Geometry check sheet. Reference: the model listing, model coordinates, mm. Face numbers are marked on the shaded views. Give positions to 0.01 mm unless a question says otherwise; leave off trailing zeros. Order: outer loops, then holes, each group sorted by start corner. A loop starts at its lowest first (then second) coordinate and runs counter-clockwise, first axis right, second up.
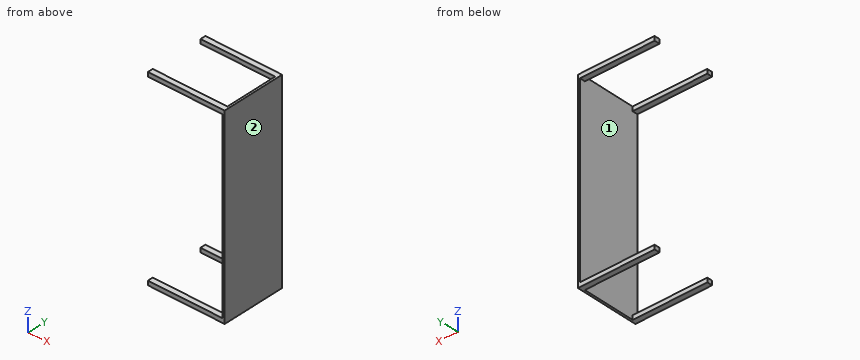
from build123d import *

# Parameters (mm, degrees)
SKETCH_1_W      = 600
SKETCH_1_H      = 1800
EXTRUDE_1_DEPTH = 20
SKETCH_2_W      = 50
SKETCH_2_H      = 40
EXTRUDE_2_DEPTH = 700


with BuildPart() as part:
    # 스케치1 → 보스-돌출1 (new body)
    with BuildSketch(Plane.YZ):
        with Locations((110.745233969, -816.291161179)):
            Rectangle(SKETCH_1_W, SKETCH_1_H)
    extrude(amount=EXTRUDE_1_DEPTH)

    # 스케치2 → 보스-돌출2 (add)
    with BuildSketch(Plane(origin=(0, 0, 0), x_dir=(0, -1, 0), z_dir=(-1, 0, 0))):
        with Locations((-385.745233969, -1696.291161179)):
            Rectangle(SKETCH_2_W, SKETCH_2_H)
        with Locations((-385.745233969, 63.708838821)):
            Rectangle(SKETCH_2_W, SKETCH_2_H)
        with Locations((164.254766031, 63.708838821)):
            Rectangle(SKETCH_2_W, SKETCH_2_H)
        with Locations((164.254766031, -1696.291161179)):
            Rectangle(SKETCH_2_W, SKETCH_2_H)
    extrude(amount=EXTRUDE_2_DEPTH)


solid = part.part
Item 1: Draft check along Z on the marked faces 1 and 2. Enter one of: released by +Z, released by -Z, zero draft, split by the parting line, or undercut.
Reported:
face 1: undercut
face 2: zero draft
Item 2: Sectioned sample at A-A (x = -47). Enter the section's corners in (y, z), and give its area (3 significant figures).
Reported:
outline: (-189.25, -1716.29) - (-139.25, -1716.29) - (-139.25, -1676.29) - (-189.25, -1676.29) - close; (-189.25, 43.71) - (-139.25, 43.71) - (-139.25, 83.71) - (-189.25, 83.71) - close; (360.75, -1716.29) - (410.75, -1716.29) - (410.75, -1676.29) - (360.75, -1676.29) - close; (360.75, 43.71) - (410.75, 43.71) - (410.75, 83.71) - (360.75, 83.71) - close
area: 8,000 mm2
Item 3: Scan lines: L1, parallel to Z at x = -615.5, y = -155; L2, parallel to X at y = 181.5, z = -1228. Record each from-to range of solid material in increasing order.
Reported:
L1: z = -1716.29 to -1676.29, 43.71 to 83.71
L2: x = 0 to 20
Item 4: Sectioned sample at B-B (z = -1299). Enter the section's corners in (x, y), and give its area (3 significant figures).
Reported:
outline: (0, -189.25) - (20, -189.25) - (20, 410.75) - (0, 410.75) - close
area: 12,000 mm2
Item 5: Sectioned sample at C-C (y = 198.5). Enter the section's corners in (x, z).
Reported:
outline: (0, -1716.29) - (20, -1716.29) - (20, 83.71) - (0, 83.71) - close
Item 6: Gauge pin test, flat end, axial feed: pin 1 (6 mm diameter, centred on y = 17, z = -600.5, fed in from -X). Record the tip position at first contact, or that the pin passes through.
Reported:
pin 1: stops at x = 0
